Read the model definition and answer for the solid it produces. Units are mm, in the model's axes. A direction names the side the tool comes from. Coordinates: 2 decimals unless noted, no trailing zeros. Order: outer loops, then holes, each group sorted by start corner. A loop starts at its lowest first (then second) coordinate and runs counter-clockwise, first axis right, second up. Notation, with made-up numbers: (49, -39) -> (75, -39) arc R17 ccw to (75, -30) -> close; hole circle Ø11 at (-17.5, 36.25). An arc over 180 degrees is marked (long way). Answer in a Markdown table with one row per item.
Autodesk Inventor part; units mm, degrees
ref_plane "YZ Plane" through (0, 0, 0) normal (1, 0, 0) x (0, 1, 0)
ref_plane "XZ Plane" through (0, 0, 0) normal (0, 1, 0) x (-1, 0, 0)
ref_plane "XY Plane" through (0, 0, 0) normal (0, 0, 1) x (1, 0, 0)
sketch "Sketch1" plane through (0, 0, 0) normal (0, 1, 0) x (-1, 0, 0)
  line L0 (0, 0) -> (5, 0)
  line L1 (5, 0) -> (5, -5)
  line L2 (5, -5) -> (0, -5)
  line L3 (0, -5) -> (0, 0)
  dimension "d0" = 5
  dimension "d1" = 5
extrude "Extrusion1" add sketch "Sketch1" along normal blind 2
sketch "Sketch3" plane through (0, 2, 0) normal (0, 1, 0) x (1, 0, 0)
  line L0 (-5, 0) -> (0, 0)
  line L1 (0, 5) -> (-5, 5)
  line L2 (0, 0) -> (-2, 0)
  line L3 (-2, 0) -> (-2, 5)
  line L4 (-2, 5) -> (0, 5)
  line L5 (0, 5) -> (0, 0)
  dimension "d4" = 2
extrude "Extrusion2" add sketch "Sketch3" along normal blind 14.5
properties part number "Knuckle Stopper - Palm"
Q1. For faces 1 (the face through (-2, 9, -2)), 2 (the face through (-1, 8, -5)), determine the directions among +Z, -Z, +X, -X, +Y, -Y from which every point of the face is accessible in a straight line to the end or side of a thin tool.
Outcome:
| item | result |
|---|---|
| face 1 | +Z, -Z, -X, +Y |
| face 2 | -Z, +X, -X, +Y, -Y |
Q2. The part is cut by section B-B (y = 15.5). Write down the section's boundary in (x, z).
Outcome:
| item | result |
|---|---|
| outline | (-2, -5) -> (0, -5) -> (0, 0) -> (-2, 0) -> close |
Q3. Given pin 1 (1.5 mm diameter, centred on x = -4, z = -3.5, fed in from +Y); pin 2 (3 mm diameter, centred on y = 4, z = -3.5, fed in from -X), each flat-ended and moving along its own axis, determine where each tip first touches the part or whether it passes through.
Outcome:
| item | result |
|---|---|
| pin 1 | y = 2 |
| pin 2 | x = -2 |
Q4. Consider line 1 (Y direction, x = -2.8, z = -1.35); line 2 (X direction, y = 11.75, z = -1.35). Determine where each line is inside the solid, lowest interval first.
Outcome:
| item | result |
|---|---|
| line 1 | 0 to 2 |
| line 2 | -2 to 0 |
Q5. The part is cut by section A-A (z = -1). Write down the section's boundary in (x, y), then the cut area to 3 significant figures.
Outcome:
| item | result |
|---|---|
| outline | (-5, 0) -> (0, 0) -> (0, 16.5) -> (-2, 16.5) -> (-2, 2) -> (-5, 2) -> close |
| area | 39.0 mm² |
Q6. The part is cut by section C-C (x = -3.9). Write down the section's boundary in (y, z).
Outcome:
| item | result |
|---|---|
| outline | (0, -5) -> (2, -5) -> (2, 0) -> (0, 0) -> close |
